Model file for the job. Use its own axes, mm. A direction names the side the tool comes from. Round coordinates to 2 decimals unless told otherwise and drop trailing zeros. Order: outer loops, then holes, each group sorted by start corner. A loop starts at its lowest first (then second) coordinate and runs counter-clockwise, first axis right, second up. Notation, with made-up numbers: (67, 68.5) -> (104, 68.5) arc R14 cw to (104, 74.5) -> close; hole circle Ø7 at (70, 4). An arc over 180 degrees is marked (long way). Put each result on its own line as item: value. Start each with the question number.
Q1. Flat gauge pins, fed straight in: P1, Ø2, axis at x = -17.5, z = -4.5, coming from the +Y side; P2, Ø3, axis at x = -26, z = -8.5, coming from the -Y side; P3, Ø3, axis at y = 4.5, z = -15, coming from the -X side. Where does each tip first touch, or does it go through?
Q2. Probe L1, parallel to Z at x = -16.75, y = 1.45; L2, parallel to X at y = 4.2, z = -12.5; L3, parallel to Z at x = -15.75, y = 2.25. List the from-to ranges inside material, lowest first.
Q3. Cut at C-C, the plane y = 3.3. List the corners of the cut face in (x, z).
Q4. Pull direction X, two halves, no side cores. Call faces 4 (the face through (-20.379, 4.287, -4.72)), 5 (the face through (-20.344, 4.248, -24.759)), 6 (the face through (-8.771, 0.713, -13.147)): released by +X, released by -X, zero draft, split by the parting line, or undercut.
Q5. 3-axis set-ups, long thin cutter, end or side, ignore diameter. For faces 1 (the face through (-28.771, 0.713, -13.112)), 2 (the face through (-20.344, 0.752, -1.185)), 3 (the face through (-12.267, 4.287, -13.112)): which of +Z, -Z, +X, -X, +Y, -Y reach the whole face in a straight line?
from build123d import *

# Parameters (mm, degrees)
SKETCH1_W           = 25
SKETCH1_H           = 25
BOSS_EXTRUDE1_DEPTH = 5
SKETCH2_W           = 15
SKETCH2_H           = 15
CUT_EXTRUDE1_DEPTH  = 5
FILLET1_R           = 2.5
FILLET2_R           = 2.5


with BuildPart() as part:
    # Sketch1 → Boss-Extrude1 (new body)
    with BuildSketch(Plane(origin=(0, 0, 0), x_dir=(1, 0, 0), z_dir=(0, 1, 0))):
        with Locations((-20.518867925, 12.971698113)):
            Rectangle(SKETCH1_W, SKETCH1_H)
    extrude(amount=BOSS_EXTRUDE1_DEPTH)

    # Sketch2 → Cut-Extrude1 (cut)
    with BuildSketch(Plane(origin=(0, 5, 0), x_dir=(1, 0, 0), z_dir=(0, 1, 0))):
        with Locations((-20.518867925, 12.971698113)):
            Rectangle(SKETCH2_W, SKETCH2_H)
    extrude(amount=-CUT_EXTRUDE1_DEPTH, mode=Mode.SUBTRACT)

    # Fillet1
    fillet1_edges = [part.edges().sort_by_distance(p)[0] for p in [
        (-20.518867925, 5, -0.471698113),
        (-33.018867925, 5, -12.971698113),
        (-28.018867925, 5, -12.971698113),
        (-20.518867925, 5, -5.471698113),
        (-13.018867925, 5, -12.971698113),
        (-20.518867925, 5, -20.471698113),
        (-20.518867925, 5, -25.471698113),
        (-8.018867925, 5, -12.971698113),
    ]]
    fillet(fillet1_edges, radius=FILLET1_R - 0.0001)  # a hair under: the kernel refuses the full size

    # Fillet2
    fillet2_edges = [part.edges().sort_by_distance(p)[0] for p in [
        (-33.018867925, 0, -12.971698113),
        (-20.518867925, 0, -0.471698113),
        (-8.018867925, 0, -12.971698113),
        (-20.518867925, 0, -25.471698113),
        (-20.518867925, 0, -20.471698113),
        (-13.018867925, 0, -12.971698113),
        (-20.518867925, 0, -5.471698113),
        (-28.018867925, 0, -12.971698113),
    ]]
    fillet(fillet2_edges, radius=FILLET2_R - 0.0001)  # a hair under: the kernel refuses the full size


solid = part.part
Ans:
1. P1: stops at y = 4.94
1. P2: passes through
1. P3: stops at x = -32.97
2. L1: z = -25.24 to -20.7, -5.24 to -0.7
2. L2: x = -32.35 to -28.69, -12.35 to -8.69
2. L3: z = -25.46 to -20.48, -5.46 to -0.48
3. outline: (-32.89, -25.34) -> (-8.15, -25.34) -> (-8.15, -0.6) -> (-32.89, -0.6) -> close; hole (-28.15, -20.6) -> (-12.89, -20.6) -> (-12.89, -5.34) -> (-28.15, -5.34) -> close
4. face 4: undercut
4. face 5: zero draft
4. face 6: released by +X
5. face 1: -Y
5. face 2: +Z, +X, -X, -Y
5. face 3: +Y
